from build123d import *

# Parameters (mm, degrees)
SKETCH2_W           = 45
SKETCH2_H           = 36.5
SKETCH2_W_2         = 32
SKETCH2_H_2         = 22.5
BOSS_EXTRUDE2_DEPTH = 22.5
SKETCH3_W           = 40
SKETCH3_H           = 22.5
CUT_EXTRUDE1_DEPTH  = 33.441832562
SKETCH5_R           = 3.25
BOSS_EXTRUDE3_DEPTH = 4
SKETCH7_R           = 3.25
CUT_EXTRUDE2_DEPTH  = 47.501639756
CUT_EXTRUDE3_START  = -18.5
SKETCH8_R           = 4.875
CUT_EXTRUDE3_DEPTH  = 18.5
FILLET1_R           = 2


with BuildPart() as part:
    # Sketch2 → Boss-Extrude2 (new body)
    with BuildSketch(Plane(origin=(0, 0, 0), x_dir=(1, 0, 0), z_dir=(0, 1, 0))):
        Rectangle(SKETCH2_W, SKETCH2_H)
        Rectangle(SKETCH2_W_2, SKETCH2_H_2, mode=Mode.SUBTRACT)
    extrude(amount=-BOSS_EXTRUDE2_DEPTH)

    # Sketch3 → Cut-Extrude1 (cut, through all)
    with BuildSketch(Plane(origin=(0, -7.9, 0), x_dir=(1, 0, 0), z_dir=(0, 1, 0))):
        Rectangle(SKETCH3_W, SKETCH3_H)
    extrude(amount=-CUT_EXTRUDE1_DEPTH, mode=Mode.SUBTRACT)

    # Sketch5 → Boss-Extrude3 (add)
    with BuildSketch(Plane(origin=(0, -22.5, 0), x_dir=(-1, 0, 0), z_dir=(0, -1, 0))):
        with BuildLine():
            Line((-24.976015549, 15.825962138), (-3.476015549, 28.125962138))
            ThreePointArc((-3.476015549, 28.125962138), (0, 29.05), (3.476015549, 28.125962138))
            Line((3.476015549, 28.125962138), (24.976015549, 15.825962138))
            ThreePointArc((24.976015549, 15.825962138), (28.325069482, 11.305129115), (27.265115511, 5.779679718))
            Line((27.265115511, 5.779679718), (21.8, -2.155957702))
            Line((21.8, -2.155957702), (15.8, -2.155957702))
            Line((15.8, -2.155957702), (15.8, 11.25))
            Line((15.8, 11.25), (-15.8, 11.25))
            Line((-15.8, 11.25), (-15.8, -2.25))
            Line((-15.8, -2.25), (-21.8, -2.25))
            Line((-21.8, -2.25), (-27.28678918, 5.811336396))
            ThreePointArc((-27.28678918, 5.811336396), (-28.320782217, 11.323826531), (-24.976015549, 15.825962138))
        make_face()
        with Locations((21.5, 9.75)):
            Circle(SKETCH5_R, mode=Mode.SUBTRACT)
        with Locations((-21.5, 9.75)):
            Circle(SKETCH5_R, mode=Mode.SUBTRACT)
        with Locations(Location((0, 22.05, 0), (0, 0, 90))):
            Circle(SKETCH5_R, mode=Mode.SUBTRACT)
    extrude(amount=-BOSS_EXTRUDE3_DEPTH)

    # Sketch7 → Cut-Extrude2 (cut, through all)
    with BuildSketch(Plane(origin=(0, -22.5, 0), x_dir=(-1, 0, 0), z_dir=(0, -1, 0))):
        with Locations(Location((-21.5, 9.75, 0), (0, 0, 90))):
            Circle(SKETCH7_R)
        with Locations(Location((0, 22.05, 0), (0, 0, 90))):
            Circle(SKETCH7_R)
        with Locations(Location((21.5, 9.75, 0), (0, 0, 90))):
            Circle(SKETCH7_R)
    extrude(amount=-CUT_EXTRUDE2_DEPTH, mode=Mode.SUBTRACT)

    # Sketch8 → Cut-Extrude3 (cut)
    with BuildSketch(Plane(origin=(0, 0, 0), x_dir=(1, 0, 0), z_dir=(0, 1, 0)).offset(CUT_EXTRUDE3_START)):
        with Locations((0, 22.05)):
            Circle(SKETCH8_R)
        with Locations((-21.5, 9.75)):
            Circle(SKETCH8_R)
        with Locations((21.5, 9.75)):
            Circle(SKETCH8_R)
    extrude(amount=CUT_EXTRUDE3_DEPTH, mode=Mode.SUBTRACT)

    # Fillet1
    # the kernel refuses this fillet: 2 mm, written as the material it takes off along each edge
    with BuildSketch(Plane(origin=(-22.5, 5, -18.25), x_dir=(1, 0, 0), z_dir=(0, -1, 0))) as fillet1_piece_1_section:
        with BuildLine():
            CenterArc((FILLET1_R, FILLET1_R), FILLET1_R, 180, 90)
            Line((0, FILLET1_R), (0, 0))
            Line((0, 0), (FILLET1_R, 0))
        make_face()
    fillet1_piece_1 = extrude(amount=32.5, mode=Mode.PRIVATE)
    fillet1_piece_1 = split(fillet1_piece_1, bisect_by=Plane(origin=(-20.691017739, -18.5, -18.244599527), z_dir=(0, 1, 0)), keep=Keep.TOP, mode=Mode.PRIVATE)
    add(fillet1_piece_1, mode=Mode.SUBTRACT)
    with BuildSketch(Plane(origin=(-22.5, 5, -18.25), x_dir=(1, 0, 0), z_dir=(0, -1, 0))) as fillet1_piece_2_section:
        with BuildLine():
            CenterArc((FILLET1_R, FILLET1_R), FILLET1_R, 180, 90)
            Line((0, FILLET1_R), (0, 0))
            Line((0, 0), (FILLET1_R, 0))
        make_face()
    fillet1_piece_2 = extrude(amount=32.5, mode=Mode.PRIVATE)
    fillet1_piece_2 = split(fillet1_piece_2, bisect_by=Plane(origin=(-21.836723919, -20.5, -17.621928978), z_dir=(-0.49657364983015595, 0, -0.8679945911665335)), keep=Keep.TOP, mode=Mode.PRIVATE)
    add(fillet1_piece_2, mode=Mode.SUBTRACT)
    with BuildSketch(Plane(origin=(22.5, 5, -18.25), x_dir=(0, 0, 1), z_dir=(0, -1, 0))) as fillet1_piece_3_section:
        with BuildLine():
            CenterArc((FILLET1_R, FILLET1_R), FILLET1_R, 180, 90)
            Line((0, FILLET1_R), (0, 0))
            Line((0, 0), (FILLET1_R, 0))
        make_face()
    fillet1_piece_3 = extrude(amount=32.5, mode=Mode.PRIVATE)
    fillet1_piece_3 = split(fillet1_piece_3, bisect_by=Plane(origin=(22.38175336, -18.5, -17.085383577), z_dir=(0, 1, 0)), keep=Keep.TOP, mode=Mode.PRIVATE)
    add(fillet1_piece_3, mode=Mode.SUBTRACT)
    with BuildSketch(Plane(origin=(22.5, 5, -18.25), x_dir=(0, 0, 1), z_dir=(0, -1, 0))) as fillet1_piece_4_section:
        with BuildLine():
            CenterArc((FILLET1_R, FILLET1_R), FILLET1_R, 180, 90)
            Line((0, FILLET1_R), (0, 0))
            Line((0, 0), (FILLET1_R, 0))
        make_face()
    fillet1_piece_4 = extrude(amount=32.5, mode=Mode.PRIVATE)
    fillet1_piece_4 = split(fillet1_piece_4, bisect_by=Plane(origin=(21.836723919, -20.5, -17.621928978), z_dir=(0.49657364983015595, 0, -0.8679945911665338)), keep=Keep.TOP, mode=Mode.PRIVATE)
    add(fillet1_piece_4, mode=Mode.SUBTRACT)
    with BuildSketch(Plane(origin=(-22.5, 5, 18.25), x_dir=(1, 0, 0), z_dir=(0, -1, 0)), Plane(origin=(22.5, 5, 18.25), x_dir=(0, 0, -1), z_dir=(0, -1, 0))) as fillet1_piece_5:
        with BuildLine():
            CenterArc((FILLET1_R, -FILLET1_R), FILLET1_R, 90, 90)
            Line((0, -FILLET1_R), (0, 0))
            Line((0, 0), (FILLET1_R, 0))
        make_face()
    extrude(amount=32.5, mode=Mode.SUBTRACT)


solid = part.part
Here's how the part is built. I have some questions about the finished solid (model axes, mm). A direction names the side the tool comes from. Give positions to 0.01 mm unless a question says otherwise; leave off trailing zeros. Order: outer loops, then holes, each group sorted by start corner. A loop starts at its lowest first (then second) coordinate and runs counter-clockwise, first axis right, second up. Notation, with made-up numbers: M -10,24.25 L 45,24.25 A24 ccw 45,56.25 Z; hole C 15.25,48 d1. An arc over 180 degrees is marked long. Answer as a JSON object with one key per item and string values. Group by question number.
1) We'd pull the mould along X, two halves only. Please class faces 5 (the cylindrical face through (17.05, -7.32, -11.74)), 6 (the flat face through (18, -7.9, 2)), 7 (the flat face through (12.24, -20.53, -23.11)), 8 (the flat face through (-2, -22.5, -13)): pulls with the +X half, pulls with the -X half, needs draft (parallel to the pull), parting line crosses it, or undercut.
2) I'm going to push flat-ended pins straight in: pin 1 Ø1 at (y, z) = (-11, 6) entering from -X; pin 2 Ø10 at (x, z) = (-22.5, -8) entering from +Y; pin 3 Ø1.2 at (y, z) = (-21.5, -3.5) entering from -X; pin 4 Ø5 at (y, z) = (-17.5, -21.5) entering from +X. Where does each tip first touch, or does it pass through?
3) Please list where these lines run through material, in increasing order: L1, parallel to X at y = -6.5, z = -9.75 (3 decimals); L2, parallel to Z at x = -5.5, y = -18. Write a range as [from, to].
4) Suppose I cut it at D-D, the plane y = -20.5. Write out the boundary of the cut face in (x, z), plus the area to 3 significant figures.
5) Suppose I cut it at A-A, the plane x = 0. Write out the boundary of the cut face in (y, z) (3 decimals), plus the area to 3 significant figures.
6) On a 3-axis mill with a long thin cutter (end or side, diameter ignored), from which of +Z, -Z, +X, -X, +Y, -Y can I reach the whole of each face in a straight line? I mean faces 1 (the cylindrical face through (-16.955, -7.324, -11.513)), 2 (the flat face through (22.5, -9, -15)), 3 (the flat face through (-22.5, -11, 6)), 4 (the flat face through (20, -15, 3)). Say none if no direction works.
7) Suppose I cut it at C-C, the plane z = -9.75. Write out the boundary of the cut face in (x, y) (3 decimals).
Results found:
{
 "1": {"face 5": "undercut", "face 6": "undercut", "face 7": "pulls with the +X half", "face 8": "needs draft"},
 "2": {"pin 1": "x = -22.5", "pin 2": "y = 0", "pin 3": "x = -26.11", "pin 4": "x = 19.06"},
 "3": {"L1": "[-16.625, -16], [16, 16.625]", "L2": "[-18.25, -11.25], [11.25, 18.25]"},
 "4": {"outline": "M -27.27,-5.78 A7 ccw -24.98,-15.83 L -22.07,-17.49 A2 ccw -20.77,-18.23 L -3.48,-28.13 A7 ccw 3.48,-28.13 L 20.77,-18.23 A2 ccw 22.07,-17.49 L 24.98,-15.83 A7 ccw 27.29,-5.81 L 22.5,1.22 L 22.5,16.25 A2 ccw 20.5,18.25 L -20.5,18.25 A2 ccw -22.5,16.25 L -22.5,1.14 Z; hole C -21.5,-9.75 d6.5; hole M -20,2.16 L -15.8,2.16 L -15.8,-11.25 L 15.8,-11.25 L 15.8,2.25 L 20,2.25 L 20,11.25 L -20,11.25 Z; hole C 0,-22.05 d6.5; hole C 21.5,-9.75 d6.5", "area": "1,140 mm²"},
 "5": {"outline": "M -22.5,-29.05 L -18.5,-29.05 L -18.5,-25.3 L -22.5,-25.3 Z; M -22.5,-18.8 L -18.5,-18.8 L -18.5,-17.175 L 0,-17.175 L 0,-11.25 L -22.5,-11.25 Z; M -22.5,11.25 L 0,11.25 L 0,18.25 L -22.5,18.25 Z", "area": "312 mm²"},
 "6": {"face 1": "+Y", "face 2": "+Z, -Z, +X, +Y", "face 3": "+Z, -X, +Y", "face 4": "none"},
 "7": {"outline": "M -28.5,-22.5 L -24.75,-22.5 L -24.75,-18.5 L -28.5,-18.5 Z; M -18.25,-22.5 L -15.8,-22.5 L -15.8,-18.5 L -18.25,-18.5 Z; M -16.625,-7.9 L -16,-7.9 L -16,0 L -16.625,0 Z; M 15.8,-22.5 L 18.25,-22.5 L 18.25,-18.5 L 15.8,-18.5 Z; M 16,-7.9 L 16.625,-7.9 L 16.625,0 L 16,0 Z; M 24.75,-22.5 L 28.5,-22.5 L 28.5,-18.5 L 24.75,-18.5 Z"}
}
